Input: part model. Units: mm. Frame: model coordinates. Face numbers are marked on the shaded views. A direction names the side the tool comes from. Give positions to 0.01 mm unless a question says otherwise; leave off trailing zeros. Loops run counter-clockwise (first coordinate to the right, second up) from the corner with the lowest first, then second, coordinate; pieces in that order, holes last. Notation, with made-up numbers: (75.5, 37) - (94.5, 37) arc R5 cw to (94.5, 46) - close; hole circle Ø7 at (79, 59.5). An arc over 180 degrees is marked (long way). Answer as a JSON object with one key per item and string values. Group by question number.
(1) Section query C-C (z = 8.5). Return loops of the section in (x, y).
(2) Access query for the marked faces 1, 2, 3 and 4. Directions: +Z, -Z, +X, -X, +Y, -Y. A direction counts if a zero-diameter tool reaches every point of the face in a straight line with its end or side. Return the directions, or none.
(3) Section query A-A (y = 10). Return loops of the section in (x, z).
(4) Pin query (flat end, axial travel): P1, Ø9, axis at x = -3, y = 8, coming from the -Z side; P2, Ø8, axis at x = 6.5, z = 9, coming from the +Y side; P3, Ø2.5, axis at x = 25.5, y = 9.5, coming from the -Z side; P4, Ø18, axis at x = 0, z = 0, coming from the -Y side. Return the tip coordinate at first contact, or that it passes through.
(5) Section query D-D (y = 20.5). Return loops of the section in (x, z).
(6) Section query B-B (x = 0). Return loops of the section in (y, z), plus the area to 3 significant figures.
(7) Mould query, pull axis Z, two halves, no side actions, for the marked faces 5, 6 and 7. Classes: +Z half, -Z half, draft (parallel to the pull), parting line (faces both ways), or undercut.
(8) Material intervals for L1, parallel to Z at x = 0, y = 7; L2, parallel to Z at x = 0, y = 19.5; L3, parallel to Y at x = -23.5, z = 30, sorted ascending.
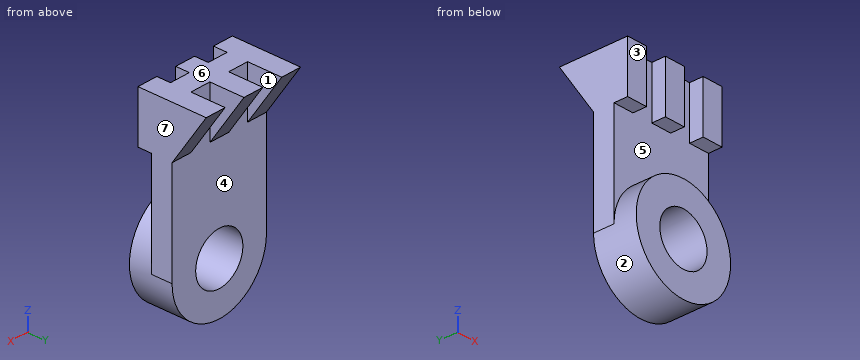
Solid Edge part; units mm, degrees
sketch "Sketch1" plane through (0, 0, 0) normal (0, -1, 0) x (1, 0, 0)
  circle A0 centre (0, 0) radius 30
  circle A1 centre (0, 0) radius 15
extrude "Protrusion1" add sketch "Sketch1" against normal blind 25
sketch "Sketch2" plane through (0, 25, 0) normal (0, 1, 0) x (0, 0, -1)
  line L0 (-90, -30) -> (-90, 30)
  line L1 (-90, 30) -> (0, 30)
  arc A0 (0, -30) -> (0, 30) centre (0, 0) cw
  line L2 (0, -30) -> (-90, -30)
extrude "ExtrudedProtrusion_2" add sketch "Sketch2" against normal blind 12
sketch "Sketch3" plane through (0, 25, 30) normal (0, 1, 0) x (0, 0, 1)
  line L0 (30, 18) -> (60, 18)
  line L1 (60, 18) -> (60, 30)
  line L2 (60, 30) -> (30, 30)
  line L3 (30, 30) -> (30, 18)
  line L4 (30, -6) -> (60, -6)
  line L5 (60, -6) -> (60, 0)
  line L6 (60, 0) -> (60, 6)
  line L7 (60, 6) -> (30, 6)
  line L8 (30, 6) -> (30, 0)
  line L9 (30, 0) -> (30, -6)
  line L10 (60, -18) -> (30, -18)
  line L11 (30, -18) -> (30, -30)
  line L12 (30, -30) -> (60, -30)
  line L13 (60, -30) -> (60, -18)
extrude "ExtrudedProtrusion_3" add sketch "Sketch3" against normal blind 20
sketch "Sketch4" plane through (-30, 15, 45) normal (-1, 0, 0) x (0, 0, 1)
  line L0 (45, 30) -> (15, 10)
  line L1 (15, 10) -> (45, 10)
  line L2 (45, 10) -> (45, 30)
extrude "ExtrudedProtrusion_4" add sketch "Sketch4" against normal blind 60
sketch "Sketch5" plane through (0, 25, 90) normal (0, 0, 1) x (0, -1, 0)
  line L0 (0, 18) -> (-20, 18)
  line L1 (-20, 18) -> (-20, 6)
  line L2 (-20, 6) -> (0, 6)
  line L3 (0, 6) -> (0, 18)
extrude "ExtrudedCutout_1" cut sketch "Sketch5" against normal blind 32
sketch "Sketch6" plane through (0, 25, 90) normal (0, 0, 1) x (0, -1, 0)
  line L0 (0, -6) -> (-20, -6)
  line L1 (-20, -6) -> (-20, -18)
  line L2 (-20, -18) -> (0, -18)
  line L3 (0, -18) -> (0, -6)
extrude "ExtrudedCutout_2" cut sketch "Sketch6" against normal blind 32
Recorded:
{
 "1": {"outline": "(-30, 13) - (-28.77, 13) - (-28.77, 0) - (-12.36, 0) - (-12.36, 25) - (-30, 25) - close; (12.36, 0) - (28.77, 0) - (28.77, 13) - (30, 13) - (30, 25) - (12.36, 25) - close"},
 "2": {"face 1": "+Z, -Z, +Y", "face 2": "-Y", "face 3": "+Z, +X, -X, -Y", "face 4": "-Z, +Y"},
 "3": {"outline": "circle Ø60 at (0, 0); (-30, 60) - (-18, 60) - (-18, 90) - (-30, 90) - close; (-6, 60) - (6, 60) - (6, 90) - (-6, 90) - close; (18, 60) - (30, 60) - (30, 90) - (18, 90) - close; hole circle Ø30 at (0, 0)"},
 "4": {"P1": "stops at z = -30", "P2": "stops at y = 25", "P3": "stops at z = -17.66", "P4": "passes through"},
 "5": {"outline": "(-30, 0) arc R30 ccw to (30, 0) - (30, 90) - (-30, 90) - close; hole circle Ø30 at (0, 0)"},
 "6": {"outline": "(0, -30) - (25, -30) - (25, -15) - (0, -15) - close; (0, 15) - (25, 15) - (25, 60) - (45, 90) - (5, 90) - (5, 60) - (13, 60) - (13, 30) - (0, 30) - close", "area": "2,010 mm^2"},
 "7": {"face 5": "undercut", "face 6": "+Z half", "face 7": "draft"},
 "8": {"L1": "z = -30 to -15, 15 to 30, 60 to 90", "L2": "z = -30 to -15, 15 to 90", "L3": "y = 13 to 25"}
}
